from build123d import *

# Parameters (mm, degrees)
F0_W     = 90
F0_H     = 885
F0_R     = 4
F1_DEPTH = 45
F2_DEPTH = 75
F3_W     = 10
F3_H     = 6
F4_DEPTH = 885


with BuildPart() as f1:
    # F0 (on Front) → F1 (new body)
    with BuildSketch(Plane.XZ):
        with Locations((540, -442.5)):
            Rectangle(F0_W, F0_H)
        Polygon((90, -885), (0, -885), (0, -975), (585, -975), (585, -885), (495, -885), align=None)
        with Locations((70, -905)):
            Circle(F0_R, mode=Mode.SUBTRACT)
        with Locations((515, -905)):
            Circle(F0_R, mode=Mode.SUBTRACT)
        with Locations((45, -442.5)):
            Rectangle(F0_W, F0_H)
        Polygon((0, 90), (0, 0), (90, 0), (495, 0), (585, 0), (585, 90), align=None)
        with Locations((70, 20)):
            Circle(F0_R, mode=Mode.SUBTRACT)
        with Locations((515, 20)):
            Circle(F0_R, mode=Mode.SUBTRACT)
    extrude(amount=F1_DEPTH)

    # F0 (on Front) → F2 (join)
    with BuildSketch(Plane.XZ):
        Polygon((90, -885), (0, -885), (0, -975), (585, -975), (585, -885), (495, -885), align=None)
        with Locations((70, -905)):
            Circle(F0_R, mode=Mode.SUBTRACT)
        with Locations((515, -905)):
            Circle(F0_R, mode=Mode.SUBTRACT)
        with Locations((45, -442.5)):
            Rectangle(F0_W, F0_H)
        with Locations((540, -442.5)):
            Rectangle(F0_W, F0_H)
    extrude(amount=F2_DEPTH)

    # F3 (on Top) → F4 (cut, through all)
    with BuildSketch(Plane.XY):
        with Locations((85, -60)):
            Rectangle(F3_W, F3_H)
    extrude(amount=-F4_DEPTH, mode=Mode.SUBTRACT)


solid = f1.part
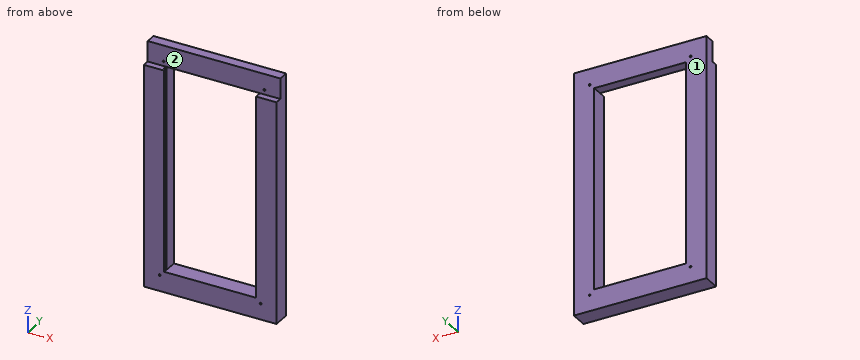
Geometry check sheet. Reference: the model listing, model coordinates, mm. Face numbers are marked on the shaded views. A direction names the side the tool comes from. Round coordinates to 2 decimals unless told otherwise and drop trailing zeros. Write each loop counter-clockwise with the first axis right and the second up, starting at its lowest first coordinate (ties: lowest second). Pieces come first, ordered by that corner, then holes.
Item 1: Section check B-B (x = 332). Record the boundary of the cut face in (y, z), plus the area to 3 significant figures.
Determined:
outline: (-75, -975) - (0, -975) - (0, -885) - (-75, -885) - close; (-45, 0) - (0, 0) - (0, 90) - (-45, 90) - close
area: 10,800 mm2
Item 2: Material ranges on line 1 along Z through (x, y) = (70, -23); line 2 along X through (y, z) = (-29, -905); line 3 along Z through (x, y) = (478, -21), recorded low to high.
Determined:
line 1: z = -975 to -909, -901 to 16, 24 to 90
line 2: x = 0 to 66, 74 to 511, 519 to 585
line 3: z = -975 to -885, 0 to 90
Item 3: Access from +Z, -Z, +X, -X, +Y, -Y to the whole of each face (thin tool, end or side, straight path). Record for the marked faces 1 and 2.
Determined:
face 1: +Z, -Z, +X, -X, +Y
face 2: +Z, +X, -X, -Y
Item 4: Section check A-A (z = -286.5). Record the boundary of the cut face in (x, y), plus the area to 3 significant figures.
Determined:
outline: (0, -75) - (90, -75) - (90, -63) - (80, -63) - (80, -57) - (90, -57) - (90, 0) - (0, 0) - close; (495, -75) - (585, -75) - (585, 0) - (495, 0) - close
area: 13,400 mm2
Item 5: Go/stop test with flat-tipped pins: pin 1 Ø24 at (x, y) = (559.5, -60) entering from +Z; pin 2 Ø10 at (x, y) = (137, -52.5) entering from +Z. Record where each tip stops, or that it passes through.
Determined:
pin 1: stops at z = 0
pin 2: stops at z = -885
